Build history of the part. All positions in model axes, mm. Face numbers are marked on the shaded views. A direction names the side the tool comes from. Coordinates: 2 decimals unless noted, no trailing zeros. Loops run counter-clockwise (first coordinate to the right, second up) from the corner with the lowest first, then second, coordinate; pieces in that order, holes last.
(1) Flat gauge pins, fed straight in: P1, Ø1.2, axis at x = -10.5, y = -37.5, coming from the -Z side; P2, Ø1, axis at x = -24, z = -1, coming from the -Y side; P3, Ø1.8, axis at x = -18, y = -34.5, coming from the -Z side. Where does each tip first touch, or does it go through?
(2) Tool access for the marked faces 4, 5 and 6: list every direction of +Z, -Z, +X, -X, +Y, -Y with a clear straight run to the whole face (end or side of a thin tool).
(3) Slice it at C-C (x = -10.5). Give the cut face in (y, z), and give its area (3 significant figures).
(4) Two-plate mould, pull along X, no slides. Class the marked faces 1, 2 and 3: pulls with the +X half, pulls with the -X half, needs draft (parallel to the pull), parting line crosses it, or undercut.
(5) Slice it at B-B (x = -20.95). Give the cut face in (y, z), and give its area (4 significant figures).
(6) Slice it at D-D (y = -3). Give the cut face in (x, z).
(7) Wall check: L1, parallel to X at y = -35.45, z = 0; L2, parallel to X at y = -35, z = 0; L3, parallel to Y at x = -3.25, z = 7. Give the ranges that are in metal, low to high.
from build123d import *

# Parameters (mm, degrees)
SKETCH1_W                 = 22.85439833
SKETCH1_H                 = 3.220407414
BOSS_EXTRUDE1_DEPTH       = 5
SKETCH2_W                 = 5
SKETCH2_H                 = 37.897484117
BOSS_EXTRUDE2_DEPTH       = 5
BOSS_EXTRUDE3_DEPTH       = 15
FILLET1_R                 = 1
BOSS_EXTRUDE28_DEPTH      = 12
BOSS_EXTRUDE28_DEPTH_BACK = 0.1
SKETCH38_W                = 12
SKETCH38_H                = 3.5
CUT_EXTRUDE3_REACH        = 47.197
SKETCH39_R                = 2.75
FILLET2_R                 = 2.5


with BuildPart() as part:
    # Sketch1 → Boss-Extrude1 (new body)
    with BuildSketch(Plane(origin=(0, 0, 0), x_dir=(0, 0, -1), z_dir=(1, 0, 0))):
        Rectangle(SKETCH1_W, SKETCH1_H)
    extrude(amount=-BOSS_EXTRUDE1_DEPTH)

    # Sketch2 → Boss-Extrude2 (add)
    with BuildSketch(Plane(origin=(0, 0, 0), x_dir=(0, 0, -1), z_dir=(1, 0, 0))):
        with Locations((0, -17.338538351)):
            Rectangle(SKETCH2_W, SKETCH2_H)
    extrude(amount=-BOSS_EXTRUDE2_DEPTH)

    # Sketch3 → Boss-Extrude3 (add)
    with BuildSketch(Plane(origin=(0, 0, 0), x_dir=(0, 0, -1), z_dir=(1, 0, 0))):
        Polygon((-9.5, -36.28728041), (-9.5, -35.28728041), (9.5, -35.28728041), (9.5, -36.28728041), (3.05, -36.28728041), (3.05, -38.68728041), (5.45, -38.68728041), (5.45, -39.68728041), (3.05, -41.28728041), (-3.05, -41.28728041), (-5.45, -39.68728041), (-5.45, -38.68728041), (-3.05, -38.68728041), (-3.05, -36.28728041), align=None)
    extrude(amount=-BOSS_EXTRUDE3_DEPTH)

    # Fillet1
    fillet1_edges = [part.edges().sort_by_distance(p)[0] for p in [
        (0, -39.18728041, 5.45),
        (0, -39.18728041, -5.45),
    ]]
    fillet(fillet1_edges, radius=FILLET1_R)

    # Sketch38 → Boss-Extrude28 (add, two sides: drawn at the far end of the back side and taken through both)
    with BuildSketch(Plane.ZY.offset(15).offset(-BOSS_EXTRUDE28_DEPTH_BACK)):
        with Locations((0, -34.53728041)):
            Rectangle(SKETCH38_W, SKETCH38_H)
    extrude(amount=BOSS_EXTRUDE28_DEPTH + BOSS_EXTRUDE28_DEPTH_BACK)

    # Sketch39 → Cut-Extrude3 (cut, up to next)
    with BuildSketch(Plane(origin=(0, -32.78728041, 0), x_dir=(1, 0, 0), z_dir=(0, 1, 0)), mode=Mode.PRIVATE) as cut_extrude3_sk1:
        with Locations(Location((-20.95, 0, 0), (0, 0, 270))):
            Circle(SKETCH39_R)
    cut_extrude3_tool1 = extrude(cut_extrude3_sk1.sketch, amount=-CUT_EXTRUDE3_REACH, mode=Mode.PRIVATE) & part.part
    add(cut_extrude3_tool1.solids().sort_by_distance((-20.95, -32.78728, 0))[0], mode=Mode.SUBTRACT)

    # Fillet2
    fillet2_edges = [part.edges().sort_by_distance(p)[0] for p in [
        (-14.9, -35.28728041, 0),
        (-15, -35.78728041, -6),
        (-15, -35.78728041, 6),
    ]]
    fillet(fillet2_edges, radius=FILLET2_R - 0.0001)  # a hair under: the kernel refuses the full size


solid = part.part
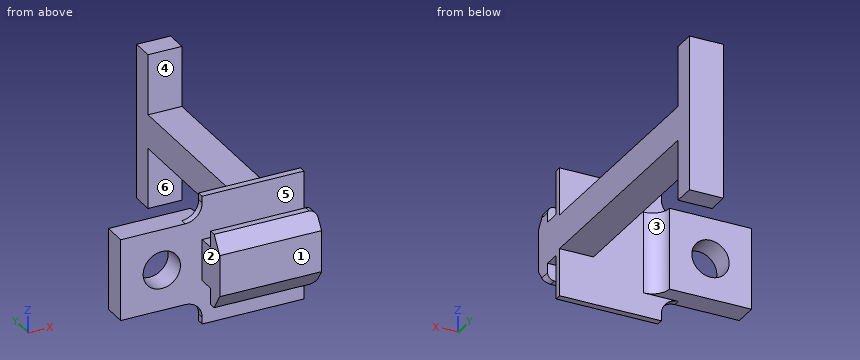
Response values:
1. P1: stops at z = -3.05
1. P2: stops at y = -36.29
1. P3: stops at z = -6
2. face 4: +Z, +X, -X
2. face 5: -X
2. face 6: -Z, +X, -X
3. outline: (-41.29, -3.05) - (-39.69, -5.45) - (-38.69, -5.45) - (-38.69, -3.05) - (-36.29, -3.05) - (-36.29, -9.5) - (-35.29, -9.5) - (-35.29, 9.5) - (-36.29, 9.5) - (-36.29, 3.05) - (-38.69, 3.05) - (-38.69, 5.45) - (-39.69, 5.45) - (-41.29, 3.05) - close
3. area: 58.1 mm2
4. face 1: needs draft
4. face 2: pulls with the -X half
4. face 3: undercut
5. outline: (-36.29, -6) - (-32.79, -6) - (-32.79, -2.75) - (-36.29, -2.75) - close; (-36.29, 2.75) - (-32.79, 2.75) - (-32.79, 6) - (-36.29, 6) - close
5. area: 22.75 mm2
6. outline: (-5, -2.5) - (0, -2.5) - (0, 2.5) - (-5, 2.5) - close
7. L1: x = -27 to -23.7, -18.2 to 0
7. L2: x = -27 to -23.7, -18.2 to -13.56, -5 to 0
7. L3: y = -36.29 to -35.29, -1.61 to 1.61
